Check sheet for the modelled part. Datum: model origin and axes. Units: mm. Face numbers are marked on the shaded views. A direction names the side the tool comes from. Give positions to 0.01 mm unless a question says otherwise; leave off trailing zeros. Loops run counter-clockwise (first coordinate to the right, second up) from the corner with the lowest first, then second, coordinate; pieces in that order, holes last. Notation, with made-up numbers: (62, 10) - (83, 10) arc R33 cw to (83, 43) - close; hole circle Ø11 at (-18.5, 89.25). An arc over 180 degrees is marked (long way). Use one line per item in the form item = value.
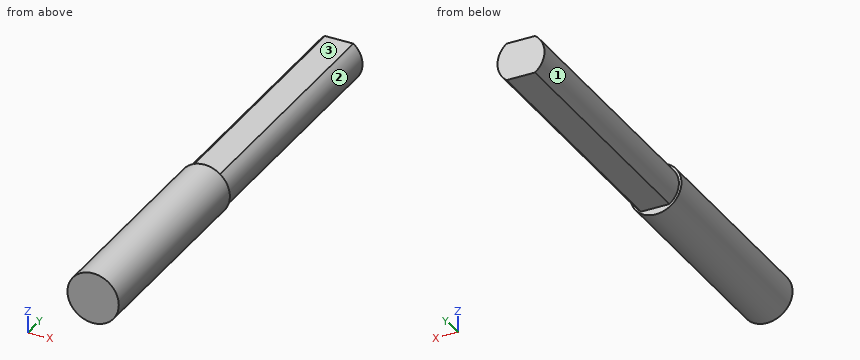
from build123d import *

# Parameters (mm, degrees)
F0_R     = 4
F1_DEPTH = 130
F2_START = 75
F0_R_2   = 7.5
F2_DEPTH = 62
F3_DEPTH = 7


with BuildPart() as f1:
    # F0 (on Front) → F1 (new body)
    with BuildSketch(Plane.XZ):
        with BuildLine():
            Line((4.2239325422, 5.5), (-4.0704200721, 5.5))
            ThreePointArc((-4.0704200721, 5.5), (-6.8423913629, 0), (-4.0704200721, -5.5))
            Line((-4.0704200721, -5.5), (4.2239325422, -5.5))
            ThreePointArc((4.2239325422, -5.5), (6.9010050788, 0), (4.2239325422, 5.5))
        make_face()
        Circle(F0_R, mode=Mode.SUBTRACT)
        Circle(F0_R)
    extrude(amount=F1_DEPTH)

    # F0 (on Front) → F2 (join)
    with BuildSketch(Plane.XZ.offset(F2_START)):
        with Locations((-0.087359423, 0)):
            Circle(F0_R_2)
        with BuildLine():
            ThreePointArc((-4.0704200721, -5.5), (-6.8423913629, 0), (-4.0704200721, 5.5))
            Line((-4.0704200721, 5.5), (4.2239325422, 5.5))
            ThreePointArc((4.2239325422, 5.5), (6.9010050788, 0), (4.2239325422, -5.5))
            Line((4.2239325422, -5.5), (-4.0704200721, -5.5))
        make_face(mode=Mode.SUBTRACT)
    extrude(amount=F2_DEPTH)

    # F3 (add): a face of the model
    f3_faces = [f1.faces().sort_by_distance(p)[0] for p in [
        (0.0391395294, -130, 0),
    ]]
    extrude(f3_faces, amount=F3_DEPTH)


solid = f1.part
Item 1: Section check B-B on x = 0.25. Record the boundary of the cut face in (y, z).
Answer block:
outline = (-137, -7.49) - (-75, -7.49) - (-75, -5.5) - (0, -5.5) - (0, 5.5) - (-75, 5.5) - (-75, 7.49) - (-137, 7.49) - close
Item 2: Section check A-A on z = 0. Record the boundary of the cut face in (x, y).
Answer block:
outline = (-7.59, -137) - (7.41, -137) - (7.41, -75) - (6.9, -75) - (6.9, 0) - (-6.84, 0) - (-6.84, -75) - (-7.59, -75) - close
Item 3: Gauge pin test, flat ends, axial feed: P1, Ø6.5, axis at x = -1, y = -45.5, coming from the -Z side; P2, Ø9, axis at x = 2, y = -32, coming from the +Z side; P3, Ø4, axis at y = -48, z = -0.5, coming from the -X side. Record the tip position at first contact, or that the pin passes through.
Answer block:
P1 = -5.5
P2 = 5.5
P3 = -6.84
Item 4: Thickness scan on L1, parallel to Z at x = 0, y = -67.5; L2, parallel to Y at x = 4, z = -6; L3, parallel to Z at x = -5.75, y = -16.5. Record the ranges inside material, lowest first.
Answer block:
L1 = -5.5 to 5.5
L2 = -137 to -75
L3 = -3.71 to 3.71
Item 5: Section check C-C on y = -114. Record the boundary of the cut face in (x, z).
Answer block:
outline = circle Ø15 at (-0.09, 0)
Item 6: Access from +Z, -Z, +X, -X, +Y, -Y to the whole of each face (thin tool, end or side, straight path). Record for the marked faces 1, 2 and 3.
Answer block:
face_1 = -X, +Y
face_2 = +X, +Y
face_3 = +Z, +X, -X, +Y
Item 7: Section check D-D on y = -28.5. Record the boundary of the cut face in (x, z).
Answer block:
outline = (-4.07, -5.5) - (4.22, -5.5) arc R6.99 ccw to (4.22, 5.5) - (-4.07, 5.5) arc R6.84 ccw to start
